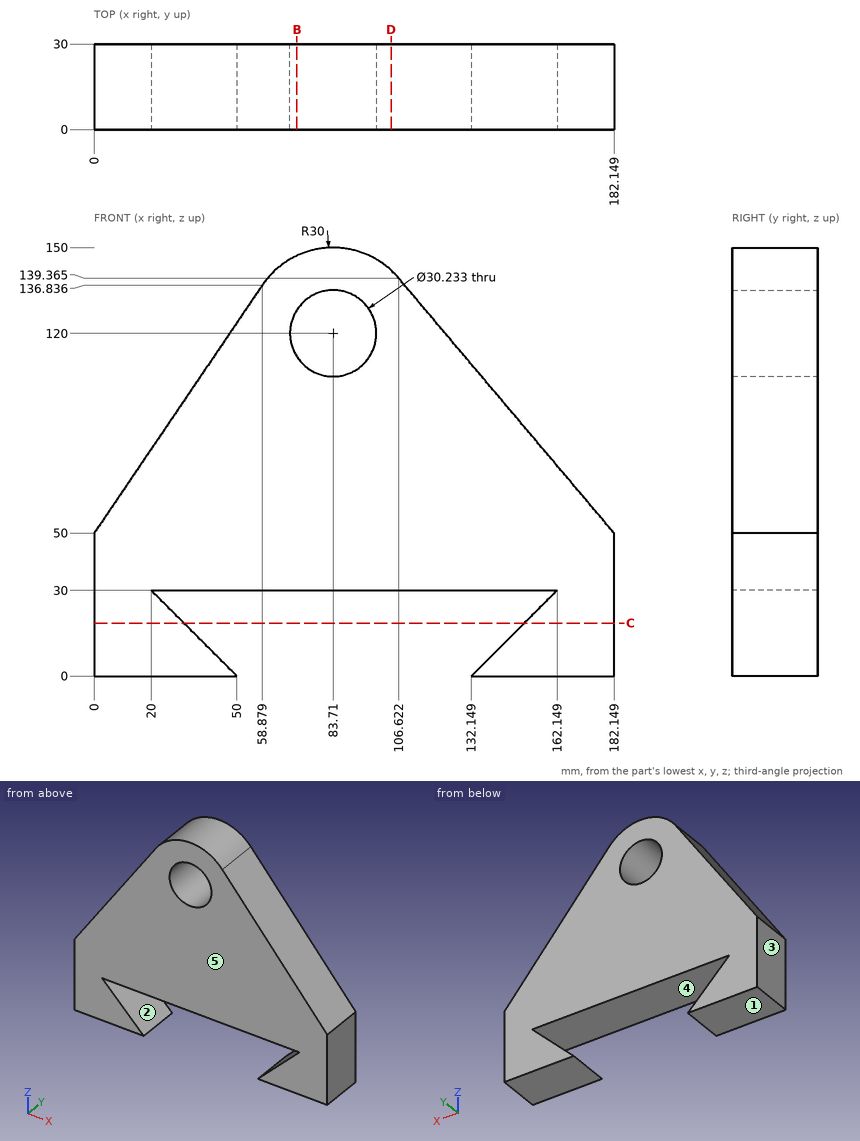
For this review, use the dimensioned drawing (mm, ordinates from the lowest corner) and the shaded views. A direction names the side the tool comes from. Round coordinates to 2 decimals unless told otherwise and drop trailing zeros. Loops run counter-clockwise (first coordinate to the right, second up) from the corner with the lowest first, then second, coordinate; pieces in that order, holes last. Notation, with made-up numbers: (43, -19) -> (65, -19) arc R30 cw to (65, 8) -> close; hole circle Ø7 at (11.25, -3.5). An arc over 180 degrees is marked (long way). Write item = value, one per line. Start each with the question number.
Item 1: Take a section at B-B on x = 71. Give the boundary of the cut face in (y, z) (1 decimal).
Item 2: Take a section at D-D on x = 104. Give the boundary of the cut face in (y, z), plus the area to 3 significant figures.
Item 3: To check wall thickness, follow L1, parallel to X at y = 19.75, z = 15.5; L2, parallel to Z at x = 22, y = 4 (1 decimal); L3, parallel to Z at x = 105, y = 12.75 (1 decimal). State the ranges of each line that lie inside material, in increasing order.
Item 4: Insertion check: pin 1 (12 mm diameter, centred on y = 24, z = 115.5, fed in from +X); pin 2 (1 mm diameter, centred on y = 4, z = 134, fed in from -X); pin 3 (3 mm diameter, centred on y = 9, z = 117, fed in from +X); pin 4 (4 mm diameter, centred on y = 8, z = 15.5, fed in from -X). Each pin has a flat end and moves straight along its axis. Give the tip position at first contact, or say it passes through.
Item 5: For the marked faces 4 and 5, list the 3-axis set-ups (+Z, -Z, +X, -X, +Y, -Y) from which the entire face can be reached by the end or side of a thin tool; tool diameter is ignored.
Item 6: Mouldability with a two-part tool opening along X and no side actions: class the marked faces 1, 2 and 3 as released by +X, released by -X, zero draft, split by the parting line, or undercut.
Item 7: Take a section at C-C on z = 18.5. Give the boundary of the cut face in (x, y).
Result:
q1.outline = (0, 30) -> (30, 30) -> (30, 111.8) -> (0, 111.8) -> close; (0, 128.2) -> (30, 128.2) -> (30, 147.2) -> (0, 147.2) -> close
q2.outline = (0, 30) -> (30, 30) -> (30, 142.1) -> (0, 142.1) -> close
q2.area = 3,360 mm²
q3.L1 = 0 to 34.5, 147.65 to 182.15
q3.L2 = 0 to 28, 30 to 82.4
q3.L3 = 30 to 141.1
q4.pin_1 = 131.86
q4.pin_2 = 56.62
q4.pin_3 = 126.79
q4.pin_4 = 0
q5.face_4 = +Y, -Y
q5.face_5 = +Z, -Z, +X, -X, -Y
q6.face_1 = zero draft
q6.face_2 = undercut
q6.face_3 = released by -X
q7.outline = (0, 0) -> (31.5, 0) -> (31.5, 30) -> (0, 30) -> close; (150.65, 0) -> (182.15, 0) -> (182.15, 30) -> (150.65, 30) -> close
